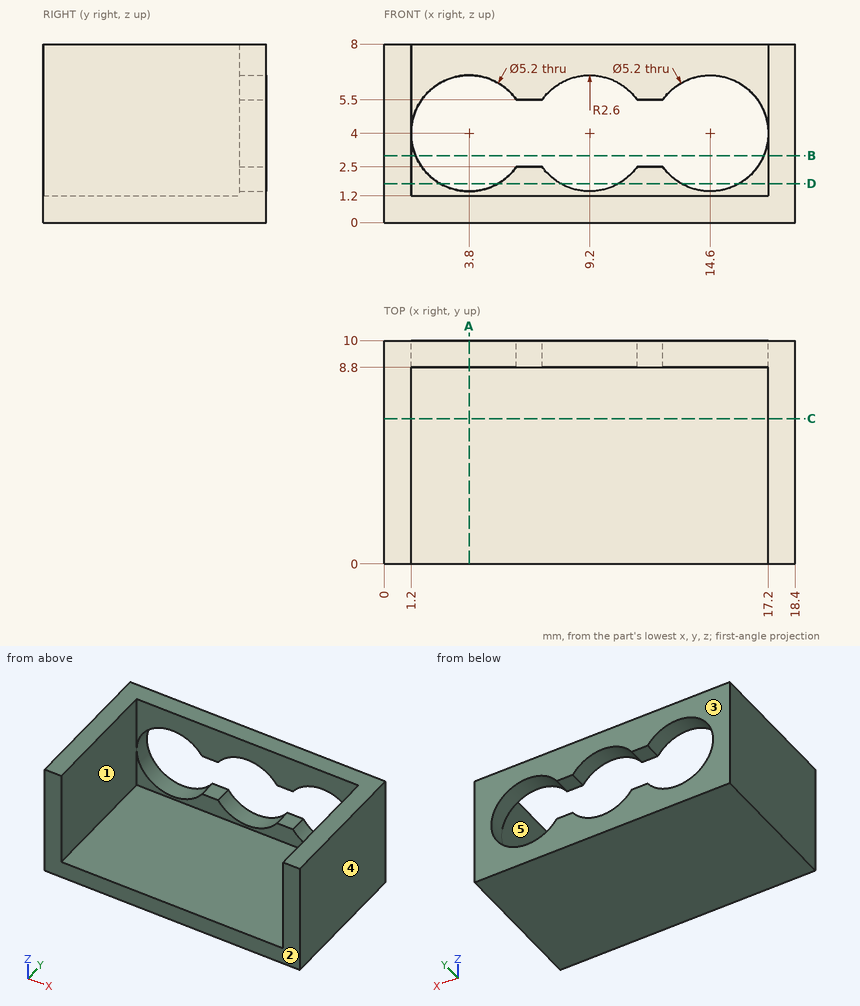
Study the drawing (mm; zero at the part's minimum x, y, z) and answer. A direction names the side the tool comes from. Give positions to 0.01 mm unless a question says otherwise; leave off trailing zeros. Write each loop counter-clockwise with the first axis right and the second up, starting at its lowest first coordinate (ties: lowest second). Pieces come first, ordered by that corner, then holes. Notation, with made-up numbers: M -35.75,24.25 L 21.25,24.25 A27 cw 21.25,46.25 Z; hole C -25.5,-26 d9. An arc over 180 degrees is marked long. Put each result on its own line as item: value. Start each with the question number.
1. The part is cut by section B-B, the plane z = 3. Give the vertices of the cut face in (x, y), and give its area (3 significant figures).
2. Consider line 1 along X through (y, z) = (5.25, 3.75); line 2 along Z through (x, y) = (3.8, 9.4); line 3 along X through (y, z) = (9.25, 1.75). Determine where each line is inside the solid, lowest interval first.
3. The part is cut by section D-D, the plane z = 1.75. Give the vertices of the cut face in (x, y).
4. For a pull along X with two mould halves and no side action, classify the marked faces 3, 4 and 5 as released by +X, released by -X, zero draft, split by the parting line, or undercut.
5. The part is cut by section C-C, the plane y = 6.5. Give the vertices of the cut face in (x, z), and give its area (3 significant figures).
6. Which of the six approach directions +Z, -Z, +X, -X, +Y, -Y give full straight-line access (tool end or side, diameter ignored) to the marked faces 1 and 2?
7. The part is cut by section A-A, the plane x = 3.8. Give the vertices of the cut face in (y, z), and give its area (3 significant figures).
8. Each of these flat-tipped pins is pushed along its axis until it touches: pin 1 Ø3 at (x, z) = (3.8, 4) entering from -Y; pin 2 Ø3 at (x, z) = (9.5, 6.5) entering from -Y. Where does it stop, or does it pass through?
Final values:
1. outline: M 0,0 L 1.2,0 L 1.2,8.8 L 1.4,8.8 L 1.4,10 L 0,10 Z; M 17,8.8 L 17.2,8.8 L 17.2,0 L 18.4,0 L 18.4,10 L 17,10 Z
1. area: 24.5 mm²
2. line 1: x = 0 to 1.2, 17.2 to 18.4
2. line 2: z = 0 to 1.4, 6.6 to 8
2. line 3: x = 0 to 2.5, 5.1 to 7.9, 10.5 to 13.3, 15.9 to 18.4
3. outline: M 0,0 L 1.2,0 L 1.2,8.8 L 2.5,8.8 L 2.5,10 L 0,10 Z; M 5.1,8.8 L 7.9,8.8 L 7.9,10 L 5.1,10 Z; M 10.5,8.8 L 13.3,8.8 L 13.3,10 L 10.5,10 Z; M 15.9,8.8 L 17.2,8.8 L 17.2,0 L 18.4,0 L 18.4,10 L 15.9,10 Z
4. face 3: zero draft
4. face 4: released by +X
4. face 5: undercut
5. outline: M 0,0 L 18.4,0 L 18.4,8 L 17.2,8 L 17.2,1.2 L 1.2,1.2 L 1.2,8 L 0,8 Z
5. area: 38.4 mm²
6. face 1: +Z, -Y
6. face 2: +Z, -Z, +X, -X, -Y
7. outline: M 0,0 L 10,0 L 10,1.4 L 8.8,1.4 L 8.8,1.2 L 0,1.2 Z; M 8.8,6.6 L 10,6.6 L 10,8 L 8.8,8 Z
7. area: 13.9 mm²
8. pin 1: passes through
8. pin 2: stops at y = 8.8
